from build123d import *

# Parameters (mm, degrees)
BOSS_EXTRUDE1_DEPTH = 5
FILLET3_R           = 0.5


with BuildPart() as part:
    # Sketch1 → Boss-Extrude1 (new body)
    with BuildSketch(Plane.XY):
        Polygon((14.1, 25.3), (14.1, 26.9), (26.1, 26.9), (26.1, 31), (24.1, 31), (24.1, 32.6), (36.1, 32.6), (36.1, 36.7), (34.1, 36.7), (34.1, 38.3), (36.1, 38.3), (36.1, 39.8), (19.3, 39.8), (19.3, 42.4), (11.3, 42.4), (11.3, 44), (16.3, 44), (16.3, 47), (-2.7, 47), (-2.7, 5), (0, 5), (0, 0), (5, 0), (5, 5), (8.5, 5), (8.5, 8), (7.4, 8), (7.4, 10.3), (8.5, 10.3), (8.5, 15), (11.5, 15), (11.5, 10.3), (12.6, 10.3), (12.6, 8), (11.5, 8), (11.5, 5), (15, 5), (15, 0), (20, 0), (20, 5), (20, 19.6), (4.1, 19.6), (4.1, 21.2), (16.1, 21.2), (16.1, 25.3), align=None)
    extrude(amount=BOSS_EXTRUDE1_DEPTH)

    # Fillet3
    fillet3_edges = [part.edges().sort_by_distance(p)[0] for p in [
        (-2.7, 47, 2.5),
        (16.3, 47, 2.5),
        (16.3, 44, 2.5),
        (19.3, 42.4, 2.5),
        (19.3, 39.8, 2.5),
        (36.1, 39.8, 2.5),
        (36.1, 38.3, 2.5),
        (36.1, 36.7, 2.5),
        (36.1, 32.6, 2.5),
        (26.1, 31, 2.5),
        (26.1, 26.9, 2.5),
        (16.1, 25.3, 2.5),
        (16.1, 21.2, 2.5),
        (20, 19.6, 2.5),
    ]]
    fillet(fillet3_edges, radius=FILLET3_R)


solid = part.part
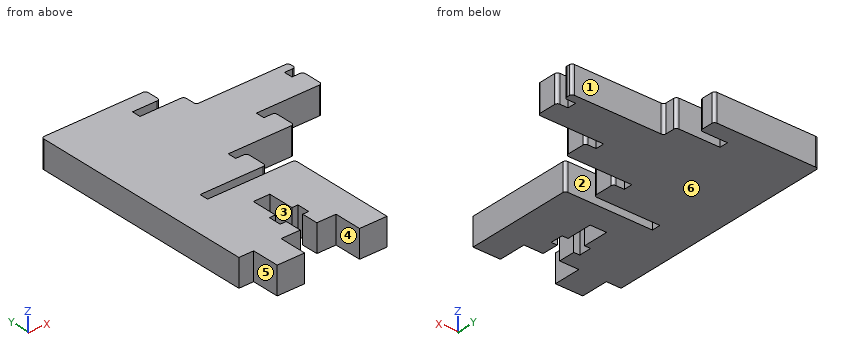
Geometry check sheet. Reference: the model listing, model coordinates, mm. Face numbers are marked on the shaded views. A direction names the side the tool comes from. Give positions to 0.01 mm unless a question says otherwise; leave off trailing zeros. Write each loop counter-clockwise with the first axis right and the second up, starting at its lowest first coordinate (ties: lowest second). Pieces come first, ordered by that corner, then holes. Notation, with made-up numbers: (-35, 27) - (9, 27) arc R17 ccw to (9, 43) - close; hole circle Ø2 at (79.25, 2.25). An arc over 180 degrees is marked (long way). Put each result on its own line as item: value.
1. Sectioned sample at A-A, the plane y = 14.5. Enter the section's corners in (x, z).
Ans:
outline: (-2.7, 0) - (8.5, 0) - (8.5, 5) - (-2.7, 5) - close; (11.5, 0) - (20, 0) - (20, 5) - (11.5, 5) - close
2. Sectioned sample at D-D, the plane y = 23. Enter the section's corners in (x, z), plus the area to 3 significant figures.
Ans:
outline: (-2.7, 0) - (16.1, 0) - (16.1, 5) - (-2.7, 5) - close
area: 94.0 mm²
3. Sectioned sample at C-C, the plane x = 22.5. Enter the section's corners in (y, z), plus the area to 3 significant figures.
Ans:
outline: (26.9, 0) - (39.8, 0) - (39.8, 5) - (26.9, 5) - close
area: 64.5 mm²
4. Thickness scan on line 1 (Y direction, x = 12.5, z = 2); line 2 (X direction, y = 11.5, z = 3.5); line 3 (X direction, y = 9, z = 1.15). Record the ranges inside material, lowest first.
Ans:
line 1: y = 5 to 8, 10.3 to 19.6, 21.2 to 42.4, 44 to 47
line 2: x = -2.7 to 8.5, 11.5 to 20
line 3: x = -2.7 to 7.4, 12.6 to 20
5. Go/stop test with flat-tipped pins: pin 1 (3 mm diameter, centred on x = 19.5, z = 4.5, fed in from +Y); pin 2 (1.5 mm diameter, centred on x = 27.5, z = 2.5, fed in from -Y); pin 3 (2.5 mm diameter, centred on x = 9.5, z = 2, fed in from -Y). Record where each tip stops, or that it passes through.
Ans:
pin 1: stops at y = 42.4
pin 2: stops at y = 32.6
pin 3: stops at y = 5
6. Sectioned sample at B-B, the plane x = 17. Enter the section's corners in (y, z), plus the area to 4 significant figures.
Ans:
outline: (0, 0) - (19.6, 0) - (19.6, 5) - (0, 5) - close; (26.9, 0) - (42.4, 0) - (42.4, 5) - (26.9, 5) - close
area: 175.5 mm²
7. Set-up check for the marked faces 1, 2 and 3: record each of +Z, -Z, +X, -X, +Y, -Y from which the full face is reachable in a straight line by a thin tool's end or side.
Ans:
face 1: +Z, -Z, +X, +Y
face 2: +Z, -Z, +X
face 3: +Z, -Z, -Y
8. Draft check along X on the marked faces 4, 5 and 6. Enter one of: +X half, -X half, draft (parallel to the pull), parting line (faces both ways), or undercut.
Ans:
face 4: undercut
face 5: -X half
face 6: draft
